Drawing for the job (mm, zero at the part's lowest x, y, z). A direction names the side the tool comes from. Give positions to 0.01 mm unless a question says otherwise; leave off trailing zeros. Order: outer loops, then holes, each group sorted by start corner. A loop starts at its lowest first (then second) coordinate and runs counter-clockwise, first axis right, second up. Notation, with made-up numbers: M 38,-14 L 93,-14 A20 ccw 93,0 Z; hole C 79,28.25 d9. An arc over 180 degrees is marked long. Answer as a JSON object with one key per item and string values.
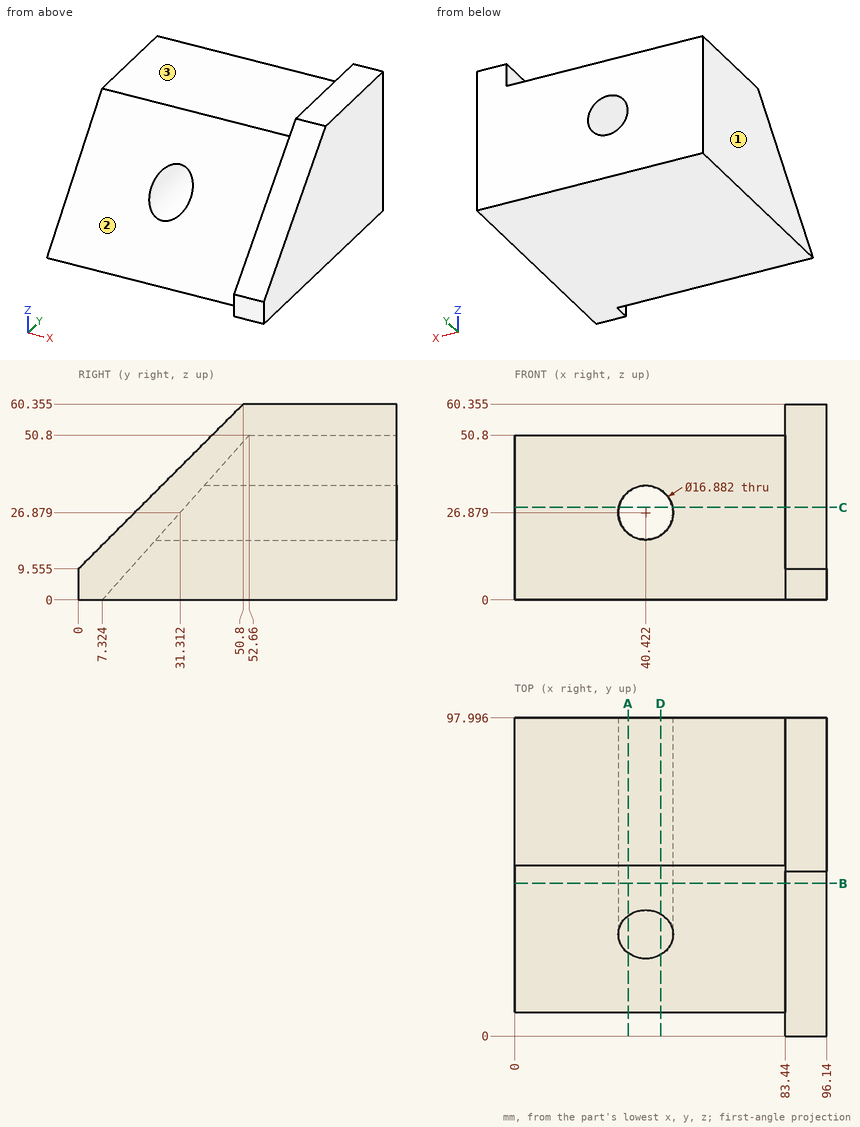
1. Cut at A-A on x = 35. Give the cut face in (y, z) (1 decimal), plus the area to 3 significant figures.
Worked answers:
{"outline": "M 7.3,0 L 98,0 L 98,20.4 L 25.5,20.4 Z; M 37.1,33.3 L 98,33.3 L 98,50.8 L 52.7,50.8 Z", "area": "2,590 mm^2"}
2. Which spindle directions (+Z, -Z, +X, -X, +Y, -Y) get a long thin tool onto all of the face, cutting with end or side? Do the marked faces 1, 2 and 3. Say none if no direction does.
Worked answers:
{"face 1": "+Z, -Z, -X, +Y, -Y", "face 2": "+Z, -X, -Y", "face 3": "+Z, -X, +Y, -Y"}
3. Probe line 1 along X through (y, z) = (41, 26.5) (1 decimal); line 2 along X through (y, z) = (37.5, 45.5); line 3 along X through (y, z) = (58, 31.5) (1 decimal). List the from-to ranges inside material, lowest first.
Worked answers:
{"line 1": "x = 0 to 32, 48.9 to 96.1", "line 2": "x = 83.44 to 96.14", "line 3": "x = 0 to 33.4, 47.5 to 96.1"}
4. Cut at C-C on z = 28.5. Give the cut face in (x, y) (1 decimal), plus the area to 3 significant figures.
Worked answers:
{"outline": "M 0,32.8 L 32.1,32.8 L 32.1,98 L 0,98 Z; M 48.7,32.8 L 83.4,32.8 L 83.4,18.9 L 96.1,18.9 L 96.1,98 L 48.7,98 Z", "area": "5,370 mm^2"}
5. Cut at D-D on x = 45. Give the cut face in (y, z).
Worked answers:
{"outline": "M 7.32,0 L 98,0 L 98,19.79 L 24.98,19.79 Z; M 37.64,33.97 L 98,33.97 L 98,50.8 L 52.66,50.8 Z"}
6. Cut at B-B on y = 47. Give the cut face in (x, z) (1 decimal), plus the area to 3 significant figures.
Worked answers:
{"outline": "M 0,0 L 96.1,0 L 96.1,56.6 L 83.4,56.6 L 83.4,44.5 L 0,44.5 Z; hole C 40.4,26.9 d16.9", "area": "4,200 mm^2"}
7. Pin check, flat tips, straight feed: P1, Ø8, axis at x = 58, y = 68, coming from the +Z side; P2, Ø1.5, axis at y = 40, z = 40.5, coming from the -X side; P3, Ø2, axis at x = 68, y = 34, coming from the +Z side. Stop position of each tip, or through.
Worked answers:
{"P1": "stops at z = 50.8", "P2": "stops at x = 83.44", "P3": "stops at z = 31.01"}
